from build123d import *

# Parameters (mm, degrees)
SKETCH_R     = 1.5
PAD_DEPTH    = 2
PAD001_DEPTH = 64


with BuildPart() as part:
    # Sketch → Pad (new body)
    with BuildSketch(Plane.XY):
        Polygon((0, 0), (30, 0), (30, 91), (-91, 91), (-91, -30), (0, -30), align=None)
        with Locations((-60, -5)):
            Circle(SKETCH_R, mode=Mode.SUBTRACT)
        with Locations((5, 60)):
            Circle(SKETCH_R, mode=Mode.SUBTRACT)
    extrude(amount=PAD_DEPTH)

    # Sketch001 (on Face9 of Pad) → Pad001 (join)
    with BuildSketch(Plane(origin=(0, 0, 0), x_dir=(1, 0, 0), z_dir=(0, 0, -1))):
        Polygon((-91, 30), (-93, 30), (-93, -93), (-91, -93), (30, -93), (30, -91), (-91, -91), align=None)
        Polygon((0, 30), (0, 0), (30, 0), (30, 2), (2, 2), (2, 30), align=None)
    extrude(amount=-PAD001_DEPTH)


solid = part.part
The listing builds one solid part. Answer for the finished solid, in the listing's coordinates (mm). A direction names the side the tool comes from. Give positions to 0.01 mm unless a question says otherwise; leave off trailing zeros. Write each loop counter-clockwise with the first axis right and the second up, starting at its lowest first coordinate (ties: lowest second). Pieces come first, ordered by that corner, then holes.
Item 1: Section B-B, the plane x = 5 is taken. Write down the section's boundary in (y, z).
Item 2: Section A-A, the plane y = -5 is taken. Write down the section's boundary in (x, z).
Item 3: Section D-D, the plane y = 60 is taken. Write down the section's boundary in (x, z).
Item 4: Section C-C, the plane x = -36.5 is taken. Write down the section's boundary in (y, z).
Item 5: Determine the mould class of faces 4 (the flat face through (-32, 31, 0)), 5 (the flat face through (-31, 31, 2)), 6 (the flat face through (-93, 31, 32)) for opening direction X: released by +X, released by -X, zero draft, split by the parting line, or undercut.
Item 6: Flat-ended cylindrical pins translate along their axes: P1, Ø14, axis at x = 20.5, z = 43.5, coming from the -Y side; P2, Ø8, axis at x = -68.5, y = 41, coming from the +Z side; P3, Ø18.5, axis at x = -38, z = 45, coming from the -Y side; P4, Ø2.5, axis at x = -60, y = -5, coming from the +Z side. Find the tip coordinate at first contact, or state that the pin passes through.
Item 7: Find the intervals of material crossed by line 1 along Y through (x, z) = (-60, 0.6); line 2 along X through (y, z) = (-17, 13); line 3 along Y through (x, z) = (6, 26.5), in increasing order.
Item 8: Which of the six approach directions +Z, -Z, +X, -X, +Y, -Y give full straight-line access (tool end or side, diameter ignored) to faces 1 (the flat face through (-30, 91, 33)), 2 (the flat face through (16, -2, 32)), 3 (the flat face through (-91, 31, 33))?
Completed:
1. outline: (-2, 0) - (58.5, 0) - (58.5, 2) - (0, 2) - (0, 64) - (-2, 64) - close; (61.5, 0) - (93, 0) - (93, 64) - (91, 64) - (91, 2) - (61.5, 2) - close
2. outline: (-93, 0) - (-61.5, 0) - (-61.5, 2) - (-91, 2) - (-91, 64) - (-93, 64) - close; (-58.5, 0) - (2, 0) - (2, 64) - (0, 64) - (0, 2) - (-58.5, 2) - close
3. outline: (-93, 0) - (3.5, 0) - (3.5, 2) - (-91, 2) - (-91, 64) - (-93, 64) - close; (6.5, 0) - (30, 0) - (30, 2) - (6.5, 2) - close
4. outline: (-30, 0) - (93, 0) - (93, 64) - (91, 64) - (91, 2) - (-30, 2) - close
5. face 4: zero draft
5. face 5: undercut
5. face 6: released by -X
6. P1: stops at y = -2
6. P2: stops at z = 2
6. P3: stops at y = 91
6. P4: passes through
7. line 1: y = -30 to -6.5, -3.5 to 93
7. line 2: x = -93 to -91, 0 to 2
7. line 3: y = -2 to 0, 91 to 93
8. face 1: +Z, +X
8. face 2: +Z, -Z, +X, -Y
8. face 3: +Z, -Y
